from build123d import *

# Parameters (mm, degrees)
CROQUIS1_W                   = 700
CROQUIS1_H                   = 50
CROQUIS1_W_2                 = 50
CROQUIS1_H_2                 = 250
CROQUIS1_H_3                 = 350
CROQUIS1_R                   = 10
SALIENTE_EXTRUIR1_DEPTH      = 450
CROQUIS4_W                   = 400
CROQUIS4_H                   = 470
CROQUIS4_H_2                 = 180
CORTAR_EXTRUIR1_DEPTH        = 151
CORTAR_EXTRUIR1_DEPTH_BACK   = 851
CROQUIS5_W                   = 30
CROQUIS5_H                   = 50
SALIENTE_EXTRUIR2_DEPTH      = 425
CROQUIS6_W                   = 15
CROQUIS6_H                   = 20
SALIENTE_EXTRUIR3_DEPTH      = 400
SALIENTE_EXTRUIR3_DEPTH_BACK = 400


with BuildPart() as part:
    # Croquis1 → Saliente-Extruir1 (new body)
    with BuildSketch(Plane.XY):
        with Locations((0, 325)):
            Rectangle(CROQUIS1_W, CROQUIS1_H)
        with Locations((325, 175)):
            Rectangle(CROQUIS1_W_2, CROQUIS1_H_2)
        with Locations((-325, 175)):
            Rectangle(CROQUIS1_W_2, CROQUIS1_H_2)
        with Locations((-325, -175)):
            Rectangle(CROQUIS1_W_2, CROQUIS1_H_3)
        with Locations((325, -175)):
            Rectangle(CROQUIS1_W_2, CROQUIS1_H_3)
        Polygon((-500, 50), (-500, 0), (-350, 0), (-300, 0), (300, 0), (350, 0), (500, 0), (500, 50), (350, 50), (300, 50), (-300, 50), (-350, 50), align=None)
        with Locations((-425, 25)):
            Circle(CROQUIS1_R, mode=Mode.SUBTRACT)
        with Locations((425, 25)):
            Circle(CROQUIS1_R, mode=Mode.SUBTRACT)
    extrude(amount=SALIENTE_EXTRUIR1_DEPTH)

    # Croquis4 → Cortar-Extruir1 (cut, two sides)
    with BuildSketch(Plane.ZY.offset(350)) as cortar_extruir1_sk:
        with Locations((225, 115)):
            Rectangle(CROQUIS4_W, CROQUIS4_H)
        with Locations((225, -260)):
            Rectangle(CROQUIS4_W, CROQUIS4_H_2)
    extrude(amount=CORTAR_EXTRUIR1_DEPTH, mode=Mode.SUBTRACT)
    extrude(cortar_extruir1_sk.sketch, amount=-CORTAR_EXTRUIR1_DEPTH_BACK, mode=Mode.SUBTRACT)

    # Croquis5 → Saliente-Extruir2 (add)
    with BuildSketch(Plane.XY.offset(450)):
        with Locations((-485, 25)):
            Rectangle(CROQUIS5_W, CROQUIS5_H)
        with Locations((485, 25)):
            Rectangle(CROQUIS5_W, CROQUIS5_H)
    extrude(amount=-SALIENTE_EXTRUIR2_DEPTH)

    # Croquis6 → Saliente-Extruir3 (add, two sides)
    with BuildSketch(Plane(origin=(0, 0, 0), x_dir=(0, 0, -1), z_dir=(1, 0, 0))) as saliente_extruir3_sk:
        with Locations((-32.5, 28.5)):
            Rectangle(CROQUIS6_W, CROQUIS6_H)
        with Locations((-417.5, 28.5)):
            Rectangle(CROQUIS6_W, CROQUIS6_H)
    extrude(amount=SALIENTE_EXTRUIR3_DEPTH)
    extrude(saliente_extruir3_sk.sketch, amount=-SALIENTE_EXTRUIR3_DEPTH_BACK)


solid = part.part
Geometry check sheet. Reference: the model listing, model coordinates, mm. A direction names the side the tool comes from. Give positions to 0.01 mm unless a question says otherwise; leave off trailing zeros. Loops run counter-clockwise (first coordinate to the right, second up) from the corner with the lowest first, then second, coordinate; pieces in that order, holes last. Notation, with made-up numbers: (-11.5, 18.25) -> (1.5, 18.25) arc R19 cw to (1.5, 46.25) -> close; hole circle Ø11 at (15.5, 45.5). An arc over 180 degrees is marked (long way). Answer in a Markdown table with one row per item. Add a question column.
1) Cross-section at C-C on y = -249. Record the boundary of the cut face in (x, z).
2) Material ranges on probe 1 along X at (y, z) = (25, 10); probe 2 along Y at (x, z) = (-425, 435.5); probe 3 along Z at (x, y) = (349.5, -202.5), recorded low to high. Write a range as from..to.
3) Set-up check for faces 5 (the face through (-4, 0, 12)), 6 (the face through (300, 173, 437)), 7 (the face through (350, 198, 437)), 8 (the face through (470, 25, 228)): record each of +Z, -Z, +X, -X, +Y, -Y from which the full face is reachable in a straight line by a thin tool's end or side.
4) Gauge pin test, flat ends, axial feed: P1, Ø2, axis at x = 351.5, z = 203, coming from the +Y side; P2, Ø7.5, axis at y = 217.5, z = 437.5, coming from the +X side; P3, Ø12.5, axis at y = 140.5, z = 10, coming from the -X side; P4, Ø16.5, axis at x = -98, z = 29, coming from the -Y side. Record the tip position at first contact, or that the pin passes through.
5) Cross-section at A-A on x = 202. Record the boundary of the cut face in (y, z), and give its area (3 significant figures).
6) Draft check along X on faces 1 (the face through (-350, 202, 12)), 2 (the face through (-7, 7, 425)), 3 (the face through (4, 50, 437)), 4 (the face through (-325, -120, 222)). Enter one of: pulls with the +X half, pulls with the -X half, needs draft (parallel to the pull), parting line crosses it, or undercut.
7) Cross-section at B-B on z = 143. Record the boundary of the cut face in (x, y), and give its area (3 significant figures).
Outcome:
| question | item | result |
|---|---|---|
| 1 | outline | (-350, 0) -> (-300, 0) -> (-300, 25) -> (-350, 25) -> close; (-350, 425) -> (-300, 425) -> (-300, 450) -> (-350, 450) -> close; (300, 0) -> (350, 0) -> (350, 25) -> (300, 25) -> close; (300, 425) -> (350, 425) -> (350, 450) -> (300, 450) -> close |
| 2 | probe 1 | x = -500..-435, -415..415, 435..500 |
| 2 | probe 2 | y = 0..15, 35..50 |
| 2 | probe 3 | z = 0..25, 425..450 |
| 3 | face 5 | +Z, -Z, -Y |
| 3 | face 6 | +Z, -Z |
| 3 | face 7 | +Z, -Z, +X, +Y |
| 3 | face 8 | +Y, -Y |
| 4 | P1 | passes through |
| 4 | P2 | stops at x = 350 |
| 4 | P3 | stops at x = -350 |
| 4 | P4 | stops at y = 0 |
| 5 | outline | (0, 0) -> (50, 0) -> (50, 25) -> (38.5, 25) -> (38.5, 40) -> (18.5, 40) -> (18.5, 25) -> (0, 25) -> close; (0, 425) -> (18.5, 425) -> (18.5, 410) -> (38.5, 410) -> (38.5, 425) -> (50, 425) -> (50, 450) -> (0, 450) -> close; (300, 0) -> (350, 0) -> (350, 25) -> (300, 25) -> close; (300, 425) -> (350, 425) -> (350, 450) -> (300, 450) -> close |
| 5 | area | 5,600 mm^2 |
| 6 | face 1 | pulls with the -X half |
| 6 | face 2 | undercut |
| 6 | face 3 | undercut |
| 6 | face 4 | needs draft |
| 7 | outline | (-500, 0) -> (-470, 0) -> (-470, 50) -> (-500, 50) -> close; (-350, -170) -> (-300, -170) -> (-300, -120) -> (-350, -120) -> close; (300, -170) -> (350, -170) -> (350, -120) -> (300, -120) -> close; (470, 0) -> (500, 0) -> (500, 50) -> (470, 50) -> close |
| 7 | area | 8,000 mm^2 |
